Autodesk Inventor part; units mm, degrees
ref_plane "YZ Plane" through (0, 0, 0) normal (1, 0, 0) x (0, 1, 0)
ref_plane "XZ Plane" through (0, 0, 0) normal (0, 1, 0) x (-1, 0, 0)
ref_plane "XY Plane" through (0, 0, 0) normal (0, 0, 1) x (1, 0, 0)
sketch "Sketch1" plane through (0, 0, 0) normal (0, 1, 0) x (-1, 0, 0)
  circle A0 centre (0, 0) radius 13.5
  circle A1 centre (0, 0) radius 14.5 construction
  circle A2 centre (28, 0) radius 13.5
  circle A3 centre (28, 0) radius 14.5 construction
  circle A4 centre (56, 0) radius 13.5
  circle A5 centre (56, 0) radius 14.5 construction
  circle A6 centre (84, 0) radius 13.5
  circle A7 centre (84, 0) radius 14.5 construction
  circle A8 centre (14, 24.2487) radius 13.5
  circle A9 centre (42, 24.2487) radius 13.5
  circle A10 centre (70, 24.2487) radius 13.5
  circle A11 centre (70, -24.2487) radius 13.5
  circle A12 centre (42, -24.2487) radius 13.5
  circle A13 centre (14, -24.2487) radius 13.5
  line L0 (84, 0) -> (56, 0) construction
  circle A14 centre (14, 24.2487) radius 14.5 construction
  circle A15 centre (42, 24.2487) radius 14.5 construction
  circle A16 centre (70, 24.2487) radius 14.5 construction
  circle A17 centre (70, -24.2487) radius 14.5 construction
  circle A18 centre (42, -24.2487) radius 14.5 construction
  circle A19 centre (14, -24.2487) radius 14.5 construction
  circle A20 centre (0, 0) radius 15.5 construction
  circle A21 centre (14, 24.2487) radius 15.5 construction
  circle A22 centre (42, 24.2487) radius 15.5 construction
  circle A23 centre (70, 24.2487) radius 15.5 construction
  circle A24 centre (70, -24.2487) radius 15.5 construction
  circle A25 centre (42, -24.2487) radius 15.5 construction
  circle A26 centre (14, -24.2487) radius 15.5 construction
  arc A27 (1.2391, 15.4504) -> (1.2391, -15.4504) centre (0, 0) ccw
  arc A28 (28, 30.9008) -> (1.2391, 15.4504) centre (14, 24.2487) ccw
  arc A29 (56, 30.9008) -> (28, 30.9008) centre (42, 24.2487) ccw
  line L1 (70, 24.2487) -> (14, 24.2487) construction
  line L2 (14, 24.2487) -> (14, -24.2487) construction
  line L3 (14, -24.2487) -> (70, -24.2487) construction
  line L4 (70, -24.2487) -> (70, 24.2487) construction
  circle A30 centre (84, 0) radius 15.5 construction
  arc A31 (82.7609, 15.4504) -> (56, 30.9008) centre (70, 24.2487) ccw
  arc A32 (82.7609, -15.4504) -> (82.7609, 15.4504) centre (84, 0) ccw
  arc A33 (56, -30.9008) -> (82.7609, -15.4504) centre (70, -24.2487) ccw
  arc A34 (28, -30.9008) -> (56, -30.9008) centre (42, -24.2487) ccw
  arc A35 (1.2391, -15.4504) -> (28, -30.9008) centre (14, -24.2487) ccw
  dimension "d0" = 27
  dimension "d1" = 29
  dimension "d2" = 27
  dimension "d3" = 29
  dimension "d4" = 27
  dimension "d5" = 29
  dimension "d6" = 27
  dimension "d7" = 29
  dimension "d8" = 27
  dimension "d9" = 27
  dimension "d10" = 27
  dimension "d11" = 27
  dimension "d12" = 27
  dimension "d13" = 27
  dimension "d14" = 29
  dimension "d15" = 29
  dimension "d16" = 29
  dimension "d17" = 29
  dimension "d18" = 29
  dimension "d19" = 29
  dimension "d20" = 31
  dimension "d21" = 31
  dimension "d22" = 31
  dimension "d23" = 31
  dimension "d24" = 31
  dimension "d25" = 31
  dimension "d26" = 31
  dimension "d27" = 31
extrude "Extrusion1" add sketch "Sketch1" along normal blind 15
sketch "Sketch2" plane through (0, 15, 0) normal (0, 1, 0) x (1, 0, 0)
  arc A0 (-1.2391, 15.4504) -> (-28, 30.9008) centre (-14, 24.2487) ccw
  arc A1 (-28, 30.9008) -> (-56, 30.9008) centre (-42, 24.2487) ccw
  arc A2 (-56, 30.9008) -> (-82.7609, 15.4504) centre (-70, 24.2487) ccw
  arc A3 (-82.7609, 15.4504) -> (-82.7609, -15.4504) centre (-84, 0) ccw
  arc A4 (-82.7609, -15.4504) -> (-56, -30.9008) centre (-70, -24.2487) ccw
  arc A5 (-56, -30.9008) -> (-28, -30.9008) centre (-42, -24.2487) ccw
  arc A6 (-28, -30.9008) -> (-1.2391, -15.4504) centre (-14, -24.2487) ccw
  arc A7 (-1.2391, -15.4504) -> (-1.2391, 15.4504) centre (0, 0) ccw
  circle A8 centre (-14, 24.2487) radius 13.5
  circle A9 centre (-42, 24.2487) radius 13.5
  circle A10 centre (-70, 24.2487) radius 13.5
  circle A11 centre (-70, -24.2487) radius 13.5
  circle A12 centre (-42, -24.2487) radius 13.5
  circle A13 centre (-14, -24.2487) radius 13.5
  circle A14 centre (-84, 0) radius 13.5
  circle A15 centre (-56, 0) radius 13.5
  circle A16 centre (-28, 0) radius 13.5
  circle A17 centre (0, 0) radius 13.5
  line L0 (-116.8, -58.15) -> (36.6, -58.15)
  line L1 (36.6, -58.15) -> (36.6, 57.15)
  line L2 (36.6, 57.15) -> (-116.8, 57.15)
  line L3 (-116.8, 57.15) -> (-116.8, -58.15)
  line L4 (-116.8, -58.15) -> (36.6, 57.15) construction
  line L5 (36.6, -58.15) -> (-116.8, 57.15) construction
  arc A18 (-82.7609, 15.4504) -> (-82.7609, -15.4504) centre (-84, 0) ccw
  arc A19 (-56, 30.9008) -> (-82.7609, 15.4504) centre (-70, 24.2487) ccw
  arc A20 (-28, 30.9008) -> (-56, 30.9008) centre (-42, 24.2487) ccw
  arc A21 (-1.2391, 15.4504) -> (-28, 30.9008) centre (-14, 24.2487) ccw
  arc A22 (-1.2391, -15.4504) -> (-1.2391, 15.4504) centre (0, 0) ccw
  arc A23 (-28, -30.9008) -> (-1.2391, -15.4504) centre (-14, -24.2487) ccw
  arc A24 (-56, -30.9008) -> (-28, -30.9008) centre (-42, -24.2487) ccw
  arc A25 (-82.7609, -15.4504) -> (-56, -30.9008) centre (-70, -24.2487) ccw
  point P0 (-40.1, -0.5)
  dimension "d30" = 153.4
  dimension "d31" = 115.3
extrude "Extrusion2" add sketch "Sketch2" against normal blind 5 contours L3 L2 L1 L0
sketch "Sketch3" plane through (0, 15, 0) normal (0, 1, 0) x (1, 0, 0)
  line L0 (36.6, -58.15) -> (36.6, 57.15)
  line L1 (36.6, 57.15) -> (-116.8, 57.15)
  line L2 (-116.8, 57.15) -> (-116.8, -58.15)
  line L3 (-116.8, -58.15) -> (36.6, -58.15)
  circle A0 centre (-14, 24.2487) radius 13.5
  circle A1 centre (-42, 24.2487) radius 13.5
  circle A2 centre (-70, 24.2487) radius 13.5
  circle A3 centre (-70, -24.2487) radius 13.5
  circle A4 centre (-42, -24.2487) radius 13.5
  circle A5 centre (-14, -24.2487) radius 13.5
  circle A6 centre (-84, 0) radius 13.5
  circle A7 centre (-56, 0) radius 13.5
  circle A8 centre (-28, 0) radius 13.5
  circle A9 centre (0, 0) radius 13.5
  line L4 (-122.402, -62.3606) -> (42.202, -62.3606)
  line L5 (42.202, -62.3606) -> (42.202, 61.3606)
  line L6 (42.202, 61.3606) -> (-122.402, 61.3606)
  line L7 (-122.402, 61.3606) -> (-122.402, -62.3606)
  line L8 (-122.402, -62.3606) -> (42.202, 61.3606) construction
  line L9 (42.202, -62.3606) -> (-122.402, 61.3606) construction
  line L10 (-116.8, -58.15) -> (36.6, -58.15)
  line L11 (36.6, -58.15) -> (36.6, 57.15)
  line L12 (36.6, 57.15) -> (-116.8, 57.15)
  line L13 (-116.8, 57.15) -> (-116.8, -58.15)
  line L14 (-116.8, -58.15) -> (36.6, 57.15) construction
  line L15 (36.6, -58.15) -> (-116.8, 57.15) construction
  point P0 (-40.1, -0.5)
extrude "Extrusion3" add sketch "Sketch3" along normal blind 6 and the other way blind 3 contours L7 L6 L5 L4
sketch "Sketch4" plane through (0, 15, 0) normal (0, 1, 0) x (1, 0, 0)
  line L0 (36.6, -58.15) -> (36.6, 57.15) construction
  line L1 (36.6, 57.15) -> (-116.8, 57.15) construction
  line L2 (-116.8, 57.15) -> (-116.8, -58.15) construction
  line L3 (-116.8, -58.15) -> (36.6, -58.15) construction
  circle A0 centre (-14, 24.2487) radius 13.5 construction
  circle A1 centre (-42, 24.2487) radius 13.5 construction
  circle A2 centre (-70, 24.2487) radius 13.5 construction
  circle A3 centre (-70, -24.2487) radius 13.5 construction
  circle A4 centre (-42, -24.2487) radius 13.5 construction
  circle A5 centre (-14, -24.2487) radius 13.5 construction
  circle A6 centre (-84, 0) radius 13.5 construction
  circle A7 centre (-56, 0) radius 13.5 construction
  circle A8 centre (-28, 0) radius 13.5 construction
  circle A9 centre (0, 0) radius 13.5 construction
  line L4 (-116.8, 57.15) -> (-109.572, 57.15) construction
  line L5 (-109.572, 57.15) -> (-109.572, 25.4) construction
  line L6 (-109.572, 25.4) -> (-116.8, 25.4) construction
  line L7 (-116.8, 25.4) -> (-116.8, 57.15) construction
  line L8 (36.6, 57.15) -> (29.372, 57.15) construction
  line L9 (29.372, 57.15) -> (29.372, 25.4) construction
  line L10 (29.372, 25.4) -> (36.6, 25.4) construction
  line L11 (36.6, 25.4) -> (36.6, 57.15) construction
  line L12 (36.6, -58.15) -> (29.372, -58.15) construction
  line L13 (29.372, -58.15) -> (29.372, -26.4) construction
  line L14 (29.372, -26.4) -> (36.6, -26.4) construction
  line L15 (36.6, -26.4) -> (36.6, -58.15) construction
  line L16 (-116.8, -58.15) -> (-109.572, -58.15) construction
  line L17 (-109.572, -58.15) -> (-109.572, -26.4) construction
  line L18 (-109.572, -26.4) -> (-116.8, -26.4) construction
  line L19 (-116.8, -26.4) -> (-116.8, -58.15) construction
  circle A10 centre (-109.572, 25.4) radius 3.865
  circle A11 centre (29.372, 25.4) radius 3.365
  circle A12 centre (29.372, -26.4) radius 3.365
  circle A13 centre (-109.572, -26.4) radius 3.865
  dimension "d42" = 31.75
  dimension "d43" = 7.228
  dimension "d44" = 31.75
  dimension "d45" = 7.228
  dimension "d46" = 7.228
  dimension "d47" = 31.75
  dimension "d48" = 31.75
  dimension "d49" = 7.228
  dimension "d50" = 7.73
  dimension "d51" = 6.73
  dimension "d52" = 6.73
  dimension "d55" = 7.73
extrude "Extrusion4" cut sketch "Sketch4" against normal through all
sketch "Sketch5" plane through (-122.402, 12, 62.3606) normal (-1, 0, 0) x (0, 0, 1)
  line L0 (-77.8606, -12) -> (-77.8606, -2)
  line L1 (-46.9102, -12) -> (-46.9102, -2)
  line L2 (-119.5106, 3) -> (-4.2106, 3)
  line L3 (-123.7212, 9) -> (0, 9)
  line L4 (-77.8606, 3) -> (-46.9102, 3)
  line L5 (-46.9102, 3) -> (-46.9102, 9)
  line L6 (-46.9102, 9) -> (-77.8606, 9)
  line L7 (-77.8606, 9) -> (-77.8606, 3)
  point P0 (-62.3606, -12)
extrude "Extrusion5" cut sketch "Sketch5" against normal through all
properties part number "CELLCASE26650_3DPrint"
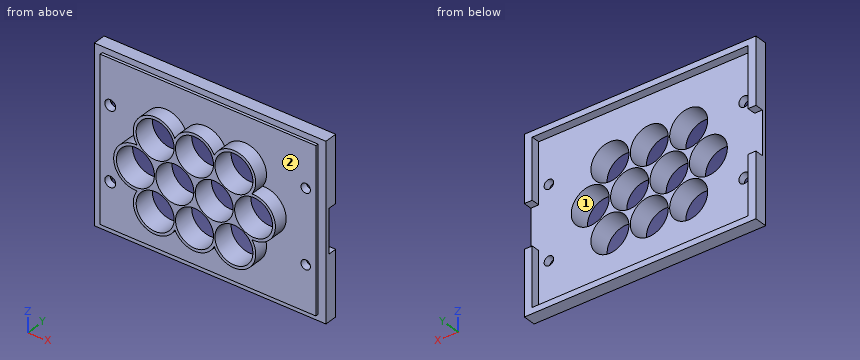
Geometry: final body of the model. Coordinates: model frame, mm. Face numbers are marked on the shaded views. A direction names the side the tool comes from. Coordinates: 2 decimals unless noted, no trailing zeros. Order: outer loops, then holes, each group sorted by start corner. A loop starts at its lowest first (then second) coordinate and runs counter-clockwise, first axis right, second up. Notation, with made-up numbers: (-25, 31.5) -> (-14, 31.5) arc R15 cw to (-14, 59.5) -> close; hole circle Ø8 at (88, 62.5). An arc over 180 degrees is marked (long way). Write each question's results on one line, items separated by ' | '. Start each with the question number.
1) Cut plane D-D, the plane z = 52. Output: boundary loops of the cut face in (x, y), and give its area (3 significant figures).
2) Cut plane C-C, the plane x = -73. Output: boundary loops of the cut face in (y, z).
3) Material intervals for line 1 along X through (y, z) = (1.5, 35.5); line 2 along Z through (x, y) = (-8.5, 8); line 3 along Z through (x, y) = (-5, 9), sorted ascending.
4) Set-up query: the marked faces 1 and 2. Return all of +Z, -Z, +X, -X, +Y, -Y with unobstructed straight access to the full face (end or side cutting, diameter ignored); none if empty.
5) Cut plane B-B, the plane y = 17.75. Output: boundary loops of the cut face in (x, z).
6) First-contact query: pin 1 (1 mm diameter, centred on x = -20.5, y = 8, fed in from +Z); pin 2 (2 mm diameter, centred on y = 8.5, z = -7, fed in from +X); pin 3 (12.5 mm diameter, centred on x = -109.572, z = 26.4, fed in from -Y). Flat tips, straight axial feed; report the tip coordinate or a pass-through.
7) Cut plane A-A, the plane z = 0. Output: boundary loops of the cut face in (x, y), and give its area (3 significant figures).
Checks:
1) outline: (-122.4, 12) -> (-116.8, 12) -> (-116.8, 10) -> (36.6, 10) -> (36.6, 12) -> (42.2, 12) -> (42.2, 21) -> (36.6, 21) -> (36.6, 15) -> (-116.8, 15) -> (-116.8, 21) -> (-122.4, 21) -> close | area: 868 mm^2
2) outline: (0, -39.46) -> (10, -39.46) -> (10, -57.15) -> (12, -57.15) -> (12, -61.36) -> (21, -61.36) -> (21, -57.15) -> (15, -57.15) -> (15, -37.41) -> (0, -37.41) -> close; (0, -11.09) -> (15, -11.09) -> (15, -7.83) -> (0, -7.83) -> close; (0, 7.83) -> (15, 7.83) -> (15, 11.09) -> (0, 11.09) -> close; (0, 37.41) -> (15, 37.41) -> (15, 58.15) -> (21, 58.15) -> (21, 62.36) -> (12, 62.36) -> (12, 58.15) -> (10, 58.15) -> (10, 39.46) -> (0, 39.46) -> close
3) line 1: -80.66 to -77.46, -62.54 to -59.34, -52.66 to -49.46, -34.54 to -31.34, -24.66 to -21.46, -6.54 to -3.34 | line 2: -38.74 to -36.58, -11.92 to -10.49, 10.49 to 11.92, 36.58 to 38.74 | line 3: -36.87 to -34.31, -14.19 to -12.54, 12.54 to 14.19, 34.31 to 36.87
4) face 1: +Y, -Y | face 2: -Y
5) outline: (-122.4, -61.36) -> (42.2, -61.36) -> (42.2, -15.5) -> (36.6, -15.5) -> (36.6, -57.15) -> (-116.8, -57.15) -> (-116.8, -15.5) -> (-122.4, -15.5) -> close; (-122.4, 15.45) -> (-116.8, 15.45) -> (-116.8, 58.15) -> (36.6, 58.15) -> (36.6, 15.45) -> (42.2, 15.45) -> (42.2, 62.36) -> (-122.4, 62.36) -> close
6) pin 1: z = 38.54 | pin 2: x = 14.29 | pin 3: y = 10
7) outline: (-122.4, 12) -> (-116.8, 12) -> (-116.8, 10) -> (-99.5, 10) -> (-99.5, 0) -> (-97.5, 0) -> (-97.5, 15) -> (-122.4, 15) -> close; (-70.5, 0) -> (-69.5, 0) -> (-69.5, 15) -> (-70.5, 15) -> close; (-42.5, 0) -> (-41.5, 0) -> (-41.5, 15) -> (-42.5, 15) -> close; (-14.5, 0) -> (-13.5, 0) -> (-13.5, 15) -> (-14.5, 15) -> close; (13.5, 0) -> (15.5, 0) -> (15.5, 10) -> (36.6, 10) -> (36.6, 12) -> (42.2, 12) -> (42.2, 15) -> (13.5, 15) -> close | area: 331 mm^2
